from build123d import *

# Parameters (mm, degrees)
BOSS_EXTRUDE1_DEPTH = 19.05
CUT_EXTRUDE1_DEPTH  = 19.05
SKETCH3_W           = 5
SKETCH3_H           = 26.05
CUT_EXTRUDE2_DEPTH  = 3


with BuildPart() as part:
    # Sketch1 → Boss-Extrude1 (new body, symmetric)
    with BuildSketch(Plane(origin=(0, 0, 0), x_dir=(0, 0, -1), z_dir=(1, 0, 0))):
        Polygon((0, 0), (-2, 0), (-2, 38), (-30, 38), (-30, 40), (0, 40), align=None)
    extrude(amount=BOSS_EXTRUDE1_DEPTH, both=True)

    # Sketch2 → Cut-Extrude1 (cut, symmetric)
    with BuildSketch(Plane(origin=(0, 40, 0), x_dir=(1, 0, 0), z_dir=(0, 1, 0))):
        with BuildLine():
            Line((11.15, -25.724165568), (11.15, -4.275834432))
            ThreePointArc((11.15, -4.275834432), (12.7, -2.725834432), (14.25, -4.275834432))
            Line((14.25, -4.275834432), (14.25, -25.724165568))
            ThreePointArc((14.25, -25.724165568), (12.7, -27.274165568), (11.15, -25.724165568))
        make_face()
        with BuildLine():
            Line((-11.15, -25.724165568), (-11.15, -4.275834432))
            ThreePointArc((-11.15, -4.275834432), (-12.7, -2.725834432), (-14.25, -4.275834432))
            Line((-14.25, -4.275834432), (-14.25, -25.724165568))
            ThreePointArc((-14.25, -25.724165568), (-12.7, -27.274165568), (-11.15, -25.724165568))
        make_face()
    extrude(amount=CUT_EXTRUDE1_DEPTH, both=True, mode=Mode.SUBTRACT)

    # Sketch3 → Cut-Extrude2 (cut, through all)
    with BuildSketch(Plane.XY.offset(2)):
        with Locations((2.5, 17.394531681)):
            Rectangle(SKETCH3_W, SKETCH3_H)
        with Locations((-2.5, 17.394531681)):
            Rectangle(SKETCH3_W, SKETCH3_H)
        with BuildLine():
            Line((-9.051280256, 30.419531681), (-9.051280256, 20.419531681))
            ThreePointArc((-9.051280256, 20.419531681), (-8.025, 19.393251425), (-6.998719744, 20.419531681))
            Line((-6.998719744, 20.419531681), (-6.998719744, 30.419531681))
            ThreePointArc((-6.998719744, 30.419531681), (-8.025, 31.445811938), (-9.051280256, 30.419531681))
        make_face()
        with BuildLine():
            Line((-9.051280256, 14.369531681), (-9.051280256, 4.369531681))
            ThreePointArc((-9.051280256, 4.369531681), (-8.025, 3.343251425), (-6.998719744, 4.369531681))
            Line((-6.998719744, 4.369531681), (-6.998719744, 14.369531681))
            ThreePointArc((-6.998719744, 14.369531681), (-8.025, 15.395811938), (-9.051280256, 14.369531681))
        make_face()
        with BuildLine():
            ThreePointArc((9.051280256, 20.419531681), (8.025, 19.393251425), (6.998719744, 20.419531681))
            Line((6.998719744, 20.419531681), (6.998719744, 30.419531681))
            ThreePointArc((6.998719744, 30.419531681), (8.025, 31.445811938), (9.051280256, 30.419531681))
            Line((9.051280256, 30.419531681), (9.051280256, 20.419531681))
        make_face()
        with BuildLine():
            ThreePointArc((9.051280256, 4.369531681), (8.025, 3.343251425), (6.998719744, 4.369531681))
            Line((6.998719744, 4.369531681), (6.998719744, 14.369531681))
            ThreePointArc((6.998719744, 14.369531681), (8.025, 15.395811938), (9.051280256, 14.369531681))
            Line((9.051280256, 14.369531681), (9.051280256, 4.369531681))
        make_face()
        Polygon((-15.786412439, 30.942427664), (-19.05, 34.716026675), (-19.05, 0), (-15.786412439, 0), align=None)
        Polygon((15.786412439, 30.942427664), (15.786412439, 0), (19.05, 0), (19.05, 34.716026675), align=None)
    extrude(amount=-CUT_EXTRUDE2_DEPTH, mode=Mode.SUBTRACT)


solid = part.part
Input: part model. Units: mm. Frame: model coordinates. A direction names the side the tool comes from. Coordinates: 2 decimals unless noted, no trailing zeros. Loops run counter-clockwise (first coordinate to the right, second up) from the corner with the lowest first, then second, coordinate; pieces in that order, holes last. Notation, with made-up numbers: (-27.75, 3) -> (-8.75, 3) arc R32 ccw to (-8.75, 39) -> close; hole circle Ø11 at (-8, -29.75). An arc over 180 degrees is marked (long way). Write each question's results on one line, items separated by ' | '. Start each with the question number.
Q1. Reachability of faces 3 (the cylindrical face through (8.048, 19.393, 1.014)), 4 (the cylindrical face through (-12.666, 39.014, 2.726)), 5 (the flat face through (0, 0, 1)), 6 (the flat face through (0, 38, 16)), 7 (the flat face through (0, 40, 15)) from +Z, -Z, +X, -X, +Y, -Y: full face, straight path, thin tool, end or side. Return the list, or none.
Q2. Pull-direction query (X, two-part tool) for faces 1 (the flat face through (0, 34, 0)), 2 (the flat face through (-9.051, 25, 1)); classes: released by +X, released by -X, zero draft, split by the parting line, or undercut.
Q3. Section D-D, the plane x = 6. Return the cut outline in (y, z).
Q4. Section C-C, the plane z = 22.5. Return the cut outline in (x, y).
Q5. Section A-A, the plane y = 24. Return the cut outline in (x, z).
Q6. Pin query (flat end, axial travel): pin 1 (0.6 mm diameter, centred on y = 24, z = 0.5, fed in from +X); pin 2 (1.5 mm diameter, centred on x = 12.5, z = 23, fed in from +Y); pin 3 (3 mm diameter, centred on x = -14.5, z = 20.5, fed in from -Y); pin 4 (2 mm diameter, centred on y = 17.5, z = 1, fed in from -X). Return the tip coordinate at first contact, or that it passes through.
Q7. Ray query, line 1 (Y direction, x = 8, z = 6.5); line 2 (Z direction, x = -9, y = 16). Return the intervals inside material, ascending. Write a range as from..to.
Q8. Section B-B, the plane x = -12.7. Return the cut outline in (y, z), plus the area to 3 significant figures.
Found:
1) face 3: +Z, -Z | face 4: +Y, -Y | face 5: +Z, -Z, +X, -X, -Y | face 6: +Z, +X, -X, -Y | face 7: +Z, -Z, +X, -X, +Y
2) face 1: zero draft | face 2: undercut
3) outline: (0, 0) -> (40, 0) -> (40, 30) -> (38, 30) -> (38, 2) -> (0, 2) -> close
4) outline: (-19.05, 38) -> (-14.25, 38) -> (-14.25, 40) -> (-19.05, 40) -> close; (-11.15, 38) -> (11.15, 38) -> (11.15, 40) -> (-11.15, 40) -> close; (14.25, 38) -> (19.05, 38) -> (19.05, 40) -> (14.25, 40) -> close
5) outline: (-15.79, 0) -> (-9.05, 0) -> (-9.05, 2) -> (-15.79, 2) -> close; (-7, 0) -> (-5, 0) -> (-5, 2) -> (-7, 2) -> close; (5, 0) -> (7, 0) -> (7, 2) -> (5, 2) -> close; (9.05, 0) -> (15.79, 0) -> (15.79, 2) -> (9.05, 2) -> close
6) pin 1: x = 15.79 | pin 2: through | pin 3: y = 38 | pin 4: x = -15.79
7) line 1: 38..40 | line 2: 0..2
8) outline: (0, 0) -> (40, 0) -> (40, 2.73) -> (38, 2.73) -> (38, 2) -> (0, 2) -> close; (38, 27.27) -> (40, 27.27) -> (40, 30) -> (38, 30) -> close | area: 86.9 mm2
